Geometry: see drawing. Coordinates: mm, zero at the bounding-box minimum. Round coordinates to 2 decimals unless told otherwise and drop trailing zeros. Write item = value, one per line. Start each with the question number.
(1) Contact query for a flat-ended pin moving along its axis: pin 1 Ø1.5 at (y, z) = (35, 3.5) entering from -X. Output: stop coordinate, or through.
(2) Ray query, line 1 (Y direction, x = 2.5, z = 3); line 2 (Y direction, x = 1.35, z = 4.5); line 3 (Z direction, x = 1.9, y = 94). Return the intervals inside material, ascending.
(3) Cut plane A-A on x = 0.6. Give the number of separate pieces and of enclosed holes in the cut face, then the cut area to 3 significant figures.
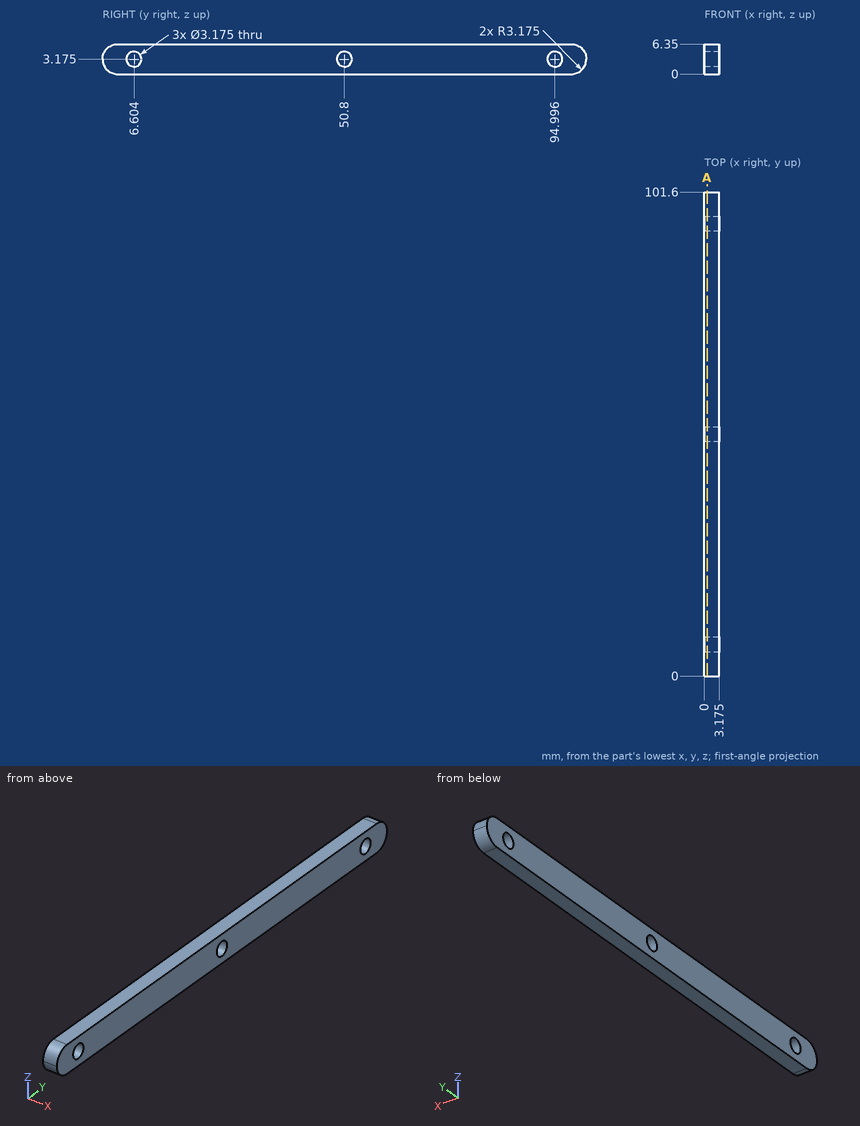
Evaluation:
q1.pin_1 = 0
q2.line_1 = 0 to 5.03, 8.18 to 49.22, 52.38 to 93.42, 96.57 to 101.6
q2.line_2 = 0.29 to 5.73, 7.48 to 49.93, 51.67 to 94.12, 95.87 to 101.31
q2.line_3 = 0 to 1.94, 4.41 to 6.35
q3.separate_pieces = 1
q3.enclosed_holes = 3
q3.area = 613 mm^2
